from build123d import *

# Parameters (mm, degrees)
SKETCH1_W           = 127.635
SKETCH1_H           = 127.635
BOSS_EXTRUDE1_DEPTH = 9.525
SKETCH13_R          = 93.6625
BOSS_EXTRUDE2_DEPTH = 9.525
SKETCH6_R           = 1.35255
F_6_32_HOLE1_DEPTH  = 12.7
SKETCH5_R           = 46.355
CUT_EXTRUDE1_DEPTH  = 9.525
SKETCH11_R          = 1.4351
CUT_EXTRUDE3_DEPTH  = 10.525
CIRPATTERN1_COUNT   = 12
SKETCH12_R          = 56.41975
CUT_EXTRUDE4_DEPTH  = 1.27


with BuildPart() as part:
    # Sketch1 → Boss-Extrude1 (new body)
    with BuildSketch(Plane(origin=(0, 0, 0), x_dir=(1, 0, 0), z_dir=(0, 1, 0))):
        with Locations((63.8175, 63.8175)):
            Rectangle(SKETCH1_W, SKETCH1_H)
    extrude(amount=BOSS_EXTRUDE1_DEPTH)

    # Sketch13 → Boss-Extrude2 (add)
    with BuildSketch(Plane(origin=(0, 9.525, 0), x_dir=(1, 0, 0), z_dir=(0, 1, 0))):
        with Locations((63.8175, 63.8175)):
            Circle(SKETCH13_R)
    extrude(amount=-BOSS_EXTRUDE2_DEPTH)

    # Sketch6 → 6-32 hole1 (cut)
    with BuildSketch(Plane(origin=(127.635, 0, 0), x_dir=(0, 0, -1), z_dir=(1, 0, 0))):
        with Locations((4.7625, 4.7625)):
            Circle(SKETCH6_R)
    extrude(amount=-F_6_32_HOLE1_DEPTH, mode=Mode.SUBTRACT)

    # Sketch5 → Cut-Extrude1 (cut)
    with BuildSketch(Plane(origin=(0, 9.525, 0), x_dir=(1, 0, 0), z_dir=(0, 1, 0))):
        with Locations((63.8175, 63.8175)):
            Circle(SKETCH5_R)
    extrude(amount=-CUT_EXTRUDE1_DEPTH, mode=Mode.SUBTRACT)

    # Sketch11 → Cut-Extrude3 (cut, through all)
    with BuildSketch(Plane(origin=(0, 9.525, 0), x_dir=(1, 0, 0), z_dir=(0, 1, 0))):
        with Locations((63.8175, 115.443)):
            Circle(SKETCH11_R)
    cut_extrude3 = extrude(amount=-CUT_EXTRUDE3_DEPTH, mode=Mode.SUBTRACT)

    # CirPattern1: Cut-Extrude3 ×12 about axis
    cirpattern1_axis = Axis((63.8175, 0, -63.8175), (0, 1, 0))
    for i in range(1, CIRPATTERN1_COUNT):
        add(cut_extrude3.rotate(cirpattern1_axis, i * 360 / CIRPATTERN1_COUNT), mode=Mode.SUBTRACT)

    # Sketch12 → Cut-Extrude4 (cut)
    with BuildSketch(Plane(origin=(0, 9.525, 0), x_dir=(1, 0, 0), z_dir=(0, 1, 0))):
        with Locations((63.8175, 63.8175)):
            Circle(SKETCH12_R)
    extrude(amount=-CUT_EXTRUDE4_DEPTH, mode=Mode.SUBTRACT)


solid = part.part
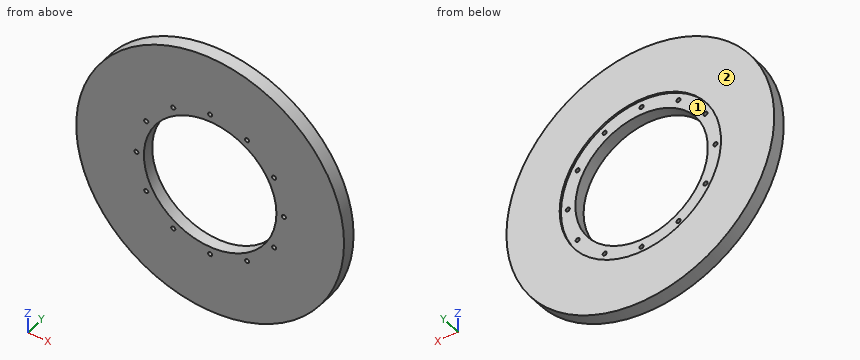
The listing builds one solid part. Answer for the finished solid, in the listing's coordinates (mm). Face numbers are marked on the shaded views. Coordinates: 2 decimals unless noted, no trailing zeros. Write each loop counter-clockwise with the first axis right and the second up, starting at its lowest first coordinate (ties: lowest second). Pieces come first, ordered by that corner, then holes. Notation, with made-up numbers: (-31, 76) - (24, 76) arc R27 ccw to (24, 114) - close; hole circle Ø7 at (36.25, 80). An arc over 180 degrees is marked (long way). Return JSON: item names as keys, results as strings.
1. The part is cut by section A-A on z = -26. Determine the outline of the cut face in (x, y) (3 decimals).
Final values:
{"outline": "(-21.871, 0) - (37.01, 0) - (37.01, 8.255) - (21.948, 8.255) - (21.948, 9.525) - (-21.871, 9.525) - close; (90.625, 0) - (149.506, 0) - (149.506, 9.525) - (105.687, 9.525) - (105.687, 8.255) - (90.625, 8.255) - close"}
2. Each of these flat-tipped pins is pushed along its axis until it touches: pin 1 Ø4 at (x, y) = (112.5, 2) entering from +Z; pin 2 Ø4 at (x, y) = (38.5, 5) entering from -Z; pin 3 Ø2 at (y, z) = (4.76, -4.76) entering from +X. Where does it stop, or does it pass through?
Final values:
{"pin 1": "z = 17.38", "pin 2": "z = -154.53", "pin 3": "x = 137.32"}
3. For a pull along X with two mould halves and no side action, classify the marked faces 1 and 2 as +X half, -X half, draft (parallel to the pull), parting line (faces both ways), or undercut.
Final values:
{"face 1": "undercut", "face 2": "draft"}
4. Consider line 1 along X through (y, z) = (7.75, -90.5); line 2 along Z through (x, y) = (104.5, 6.75); line 3 along Z through (x, y) = (51.5, 5.5). Determine where each line is inside the solid, lowest interval first.
Final values:
{"line 1": "-25.96 to 17.97, 20.25 to 25.91, 101.72 to 107.38, 109.67 to 153.6", "line 2": "-148.18 to -86.04, -41.6 to 20.55", "line 3": "-156.67 to -108.51, -19.13 to 29.03"}
5. The part is cut by section C-C on y = 1.5. Count the separate pieces of the cut face and the enclosed holes in it, then the cut area to 3 significant figures.
Final values:
{"separate pieces": "1", "enclosed holes": "13", "area": "20,700 mm^2"}
6. The part is cut by section B-B on x = 100.5. Determine the outline of the cut face in (y, z) (3 decimals).
Final values:
{"outline": "(0, -149.998) - (9.525, -149.998) - (9.525, -106.685) - (8.255, -106.685) - (8.255, -92.158) - (0, -92.158) - close; (0, -35.477) - (8.255, -35.477) - (8.255, -20.95) - (9.525, -20.95) - (9.525, 22.363) - (0, 22.363) - close"}
7. The part is cut by section D-D on x = -6. Determine the outline of the cut face in (y, z) (3 decimals), then the cut area to 3 significant figures.
Final values:
{"outline": "(0, -126.253) - (9.525, -126.253) - (9.525, -1.382) - (0, -1.382) - close", "area": "1,190 mm^2"}
